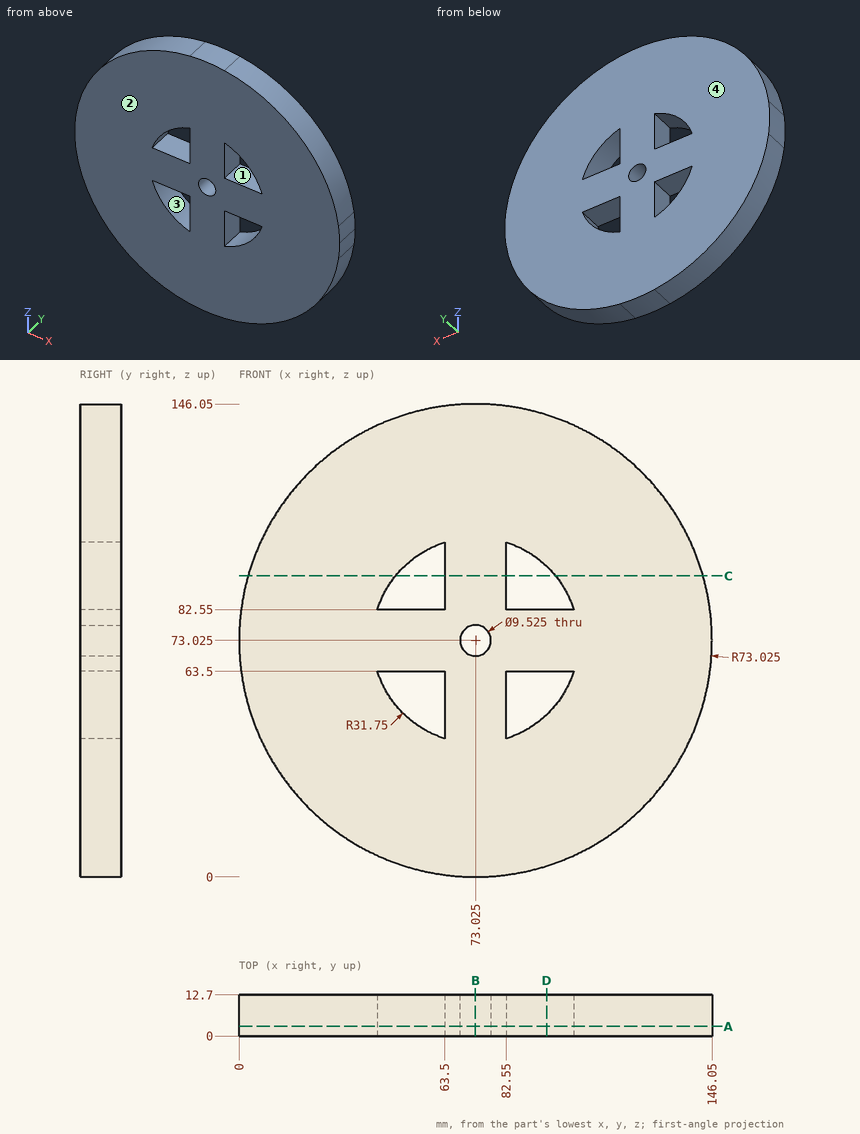
The figure shows three views and two pictorial views of one solid part (mm, origin at its lowest corner). Answer the questions. A direction names the side the tool comes from. Give positions to 0.01 mm unless a question says otherwise; leave off trailing zeros. Order: outer loops, then holes, each group sorted by start corner. A loop starts at its lowest first (then second) coordinate and runs counter-clockwise, first axis right, second up. Notation, with made-up numbers: (21.25, 76.25) -> (53.25, 76.25) arc R18 ccw to (53.25, 93.25) -> close; hole circle Ø7 at (88.25, 25). An arc over 180 degrees is marked (long way). Answer as CSV lines item,"result". Start each with the question number.
Q1. Given pin 1 (4 mm diameter, centred on x = 96.5, y = 8, fed in from +Z); pin 2 (6.5 mm diameter, centred on y = 3.5, z = 94.5, fed in from +X); pin 3 (1.5 mm diameter, centred on x = 109, y = 9, fed in from +Z); pin 4 (7.5 mm diameter, centred on x = 73.025, z = 73.025, fed in from -Y), each flat-ended and moving along its own axis, determine where each tip first touches the part or whether it passes through.
Q2. Determine the mould class of the marked faces 3 and 4 for opening direction X: pulls with the +X half, pulls with the -X half, needs draft (parallel to the pull), parting line crosses it, or undercut.
Q3. A cutting plane is placed at A-A (y = 3). Count the separate pieces of the cut face and the enclosed holes in it, then the cut area to 3 significant figures.
Q4. A cutting plane is placed at D-D (x = 95). Determine the outline of the cut face in (y, z), then the cut area to 3 significant figures.
Q5. Find the intervals of material crossed by L1, parallel to X at y = 2.25, z = 56; L2, parallel to X at y = 11.25, z = 45.5; L3, parallel to Z at x = 51, y = 3.75, in increasing order.
Q6. Which of the six approach directions +Z, -Z, +X, -X, +Y, -Y give full straight-line access (tool end or side, diameter ignored) to the marked faces 1 and 2?
Q7. A cutting plane is placed at B-B (x = 73). Determine the outline of the cut face in (y, z), then the cut area to 3 significant figures.
Q8. A cutting plane is placed at C-C (z = 93). Determine the outline of the cut face in (x, y).
Results found:
1,pin 1,"z = 142.82"
1,pin 2,"x = 143.74"
1,pin 3,"z = 136.99"
1,pin 4,"through"
2,face 3,"undercut"
2,face 4,"needs draft"
3,separate pieces,"1"
3,enclosed holes,"5"
3,area,"15,500 mm2"
4,outline,"(0, 3.38) -> (12.7, 3.38) -> (12.7, 50.11) -> (0, 50.11) -> close; (0, 63.5) -> (12.7, 63.5) -> (12.7, 82.55) -> (0, 82.55) -> close; (0, 95.94) -> (12.7, 95.94) -> (12.7, 142.67) -> (0, 142.67) -> close"
4,area,"1,430 mm2"
5,L1,"2.01 to 46.23, 63.5 to 82.55, 99.82 to 144.04"
5,L2,"5.39 to 57.2, 63.5 to 82.55, 88.85 to 140.66"
5,L3,"3.4 to 50.16, 63.5 to 82.55, 95.89 to 142.65"
6,face 1,"+Y, -Y"
6,face 2,"+Z, -Z, +X, -X, -Y"
7,outline,"(0, 0) -> (12.7, 0) -> (12.7, 68.26) -> (0, 68.26) -> close; (0, 77.79) -> (12.7, 77.79) -> (12.7, 146.05) -> (0, 146.05) -> close"
7,area,"1,730 mm2"
8,outline,"(2.79, 0) -> (48.35, 0) -> (48.35, 12.7) -> (2.79, 12.7) -> close; (63.5, 0) -> (82.55, 0) -> (82.55, 12.7) -> (63.5, 12.7) -> close; (97.7, 0) -> (143.26, 0) -> (143.26, 12.7) -> (97.7, 12.7) -> close"
